```python
from build123d import *

# Parameters (mm, degrees)
SKETCH1_R               = 2
BOSS_EXTRUDE1_DEPTH     = 20
CUT_EXTRUDE1_DEPTH      = 37.932370625
CUT_EXTRUDE1_DEPTH_BACK = 37.932370625
SKETCH2_W               = 20
SKETCH2_H               = 16.5
FILLET1_R               = 4
CHAMFER1_SIZE           = 4
CHAMFER1_SIZE_2         = 11.616843511
SKETCH4_R               = 2.5
CUT_EXTRUDE2_DEPTH      = 40.446165847
CUT_EXTRUDE3_START      = -3
CUT_EXTRUDE3_DEPTH      = 37.446165847


with BuildPart() as part:
    # Sketch1 → Boss-Extrude1 (new, symmetric)
    with BuildSketch(Plane.XY):
        with BuildLine():
            Line((-2.75862069, 2.896551724), (6.8, 12))
            Line((6.8, 12), (30, 12))
            Line((30, 12), (30, 4))
            Line((30, 4), (10, 4))
            Line((10, 4), (2.75862069, -2.896551724))
            ThreePointArc((2.75862069, -2.896551724), (-2.896551724, -2.75862069), (-2.75862069, 2.896551724))
        make_face()
        Circle(SKETCH1_R, mode=Mode.SUBTRACT)
    extrude(amount=BOSS_EXTRUDE1_DEPTH, both=True)

    # Sketch2 → Cut-Extrude1 (cut, two sides: drawn at the far end of the back side and taken through both)
    with BuildSketch(Plane.XZ.offset(-4).offset(-CUT_EXTRUDE1_DEPTH_BACK)):
        with Locations((-2, 16.75)):
            Rectangle(SKETCH2_W, SKETCH2_H)
        with Locations((-2, -16.75)):
            Rectangle(SKETCH2_W, SKETCH2_H)
    extrude(amount=CUT_EXTRUDE1_DEPTH + CUT_EXTRUDE1_DEPTH_BACK, mode=Mode.SUBTRACT)

    # Fillet1
    # the kernel refuses this fillet: 4 mm, written as the material it takes off along each edge
    with BuildSketch(Plane(origin=(8, 2.095238095, -33.4221588), x_dir=(0.7241379310344825, 0.6896551724137934, 0), z_dir=(0, 0, 1))) as fillet1_piece_1:
        with BuildLine():
            CenterArc((6.599216221, 1.129177032), FILLET1_R, 136.397181027, 60)
            Line((3.702664496, 3.887797721), (3.644733462, 3.942970135))
            Line((3.644733462, 3.942970135), (-0.057931034, 0.055172414))
            Line((-0.057931034, 0.055172414), (0, -0.08))
            ThreePointArc((0, -0.08), (1.380952381, -0.08), (2.685158533, -0.022583541))
            Line((2.685158533, -0.022583541), (2.761904762, 0))
        make_face()
    extrude(amount=24.9221588, mode=Mode.SUBTRACT)
    with BuildSketch(Plane(origin=(8, 12, -8.5), x_dir=(0, -1, 0), z_dir=(0, 0, -1))) as fillet1_piece_2:
        with BuildLine():
            CenterArc((FILLET1_R, -FILLET1_R), FILLET1_R, 90, 90)
            Line((0, -FILLET1_R), (-FILLET1_R * 0.02, -FILLET1_R))
            Line((-FILLET1_R * 0.02, -FILLET1_R), (-FILLET1_R * 0.02, FILLET1_R * 0.02))
            Line((-FILLET1_R * 0.02, FILLET1_R * 0.02), (FILLET1_R, FILLET1_R * 0.02))
            Line((FILLET1_R, FILLET1_R * 0.02), (FILLET1_R, 0))
        make_face()
    extrude(amount=21.5, mode=Mode.SUBTRACT)
    with BuildSketch(Plane(origin=(8, 12, 8.5), x_dir=(0, -1, 0), z_dir=(0, 0, 1))) as fillet1_piece_3:
        with BuildLine():
            CenterArc((FILLET1_R, FILLET1_R), FILLET1_R, 180, 90)
            Line((0, FILLET1_R), (-FILLET1_R * 0.02, FILLET1_R))
            Line((-FILLET1_R * 0.02, FILLET1_R), (-FILLET1_R * 0.02, -FILLET1_R * 0.02))
            Line((-FILLET1_R * 0.02, -FILLET1_R * 0.02), (FILLET1_R, -FILLET1_R * 0.02))
            Line((FILLET1_R, -FILLET1_R * 0.02), (FILLET1_R, 0))
        make_face()
    extrude(amount=21.5, mode=Mode.SUBTRACT)
    with BuildSketch(Plane(origin=(8, 2.095238095, 33.4221588), x_dir=(0.7241379310344824, 0.6896551724137936, 0), z_dir=(0, 0, -1))) as fillet1_piece_4:
        with BuildLine():
            CenterArc((6.599216221, -1.129177032), FILLET1_R, 163.602818973, 60)
            Line((3.702664496, -3.887797721), (3.644733462, -3.942970135))
            Line((3.644733462, -3.942970135), (-0.057931034, -0.055172414))
            Line((-0.057931034, -0.055172414), (0, 0.08))
            ThreePointArc((0, 0.08), (1.380952381, 0.08), (2.685158533, 0.022583541))
            Line((2.685158533, 0.022583541), (2.761904762, 0))
        make_face()
    extrude(amount=24.9221588, mode=Mode.SUBTRACT)

    # Chamfer1
    # the kernel refuses this chamfer: 11.616843511, 4 mm, written as the material it adds along each edge
    with BuildSketch(Plane(origin=(12, 8, -8.5), x_dir=(-1, 0, 0), z_dir=(0, -1, 0))) as chamfer1_piece_1_section:
        Polygon((4 + CHAMFER1_SIZE, 0), (4, CHAMFER1_SIZE_2), (4, 0), align=None)
    chamfer1_piece_1 = revolve(axis=Axis((12, 8, -8.5), (0, 0, -1)), revolution_arc=359.64, mode=Mode.PRIVATE)
    chamfer1_piece_1 = split(chamfer1_piece_1, bisect_by=Plane(origin=(6.815559228, 9.673675178, -20), z_dir=(0, 0, 1)), keep=Keep.TOP, mode=Mode.PRIVATE)
    chamfer1_piece_1 = split(chamfer1_piece_1, bisect_by=Plane(origin=(6.815559228, 12, -12.048091189), z_dir=(0, -1, 0)), keep=Keep.TOP, mode=Mode.PRIVATE)
    chamfer1_piece_1 = split(chamfer1_piece_1, bisect_by=Plane(origin=(5.646379541, 10.901313849, -12.048091189), z_dir=(0.6896551724137935, -0.7241379310344824, 0)), keep=Keep.TOP, mode=Mode.PRIVATE)
    chamfer1_piece_1 = split(chamfer1_piece_1, bisect_by=Plane(origin=(11.163620921, 5.1082104, -12.048091189), z_dir=(-0.6896551724137935, 0.7241379310344825, 0)), keep=Keep.TOP, mode=Mode.PRIVATE)
    add(chamfer1_piece_1)
    with BuildSketch(Plane(origin=(8, 7.464101615, -8.5), x_dir=(-0.9944459243087849, 0, 0.10524877018591122), z_dir=(0, 1, 0))) as chamfer1_piece_2_section:
        Polygon((CHAMFER1_SIZE * 0.994445924309, -CHAMFER1_SIZE * 0.105248770186), (-CHAMFER1_SIZE_2 * 0.105248770183, -CHAMFER1_SIZE_2 * 0.994445924283), (0, 0), align=None)
    chamfer1_piece_2 = extrude(amount=0.535898385, mode=Mode.PRIVATE)
    chamfer1_piece_2 = split(chamfer1_piece_2, bisect_by=Plane(origin=(6.666533122, 7.732050808, -20), z_dir=(0, 0, 1)), keep=Keep.TOP, mode=Mode.PRIVATE)
    add(chamfer1_piece_2)
    with BuildSketch(Plane(origin=(12, 7.464101615, -8.5), x_dir=(-1, 0, 0), z_dir=(0, 1, 0))) as chamfer1_piece_3_section:
        Polygon((4 + CHAMFER1_SIZE, 0), (4, -CHAMFER1_SIZE_2), (4, 0), align=None)
    chamfer1_piece_3 = revolve(axis=Axis((12, 7.464101615, -8.5), (0, 0, 1)), revolution_arc=359.64, mode=Mode.PRIVATE)
    chamfer1_piece_3 = split(chamfer1_piece_3, bisect_by=Plane(origin=(6.73533338, 5.888138527, -20), z_dir=(0, 0, 1)), keep=Keep.TOP, mode=Mode.PRIVATE)
    chamfer1_piece_3 = split(chamfer1_piece_3, bisect_by=Plane(origin=(6.73533338, 12, -12.010330429), z_dir=(0, -1, 0)), keep=Keep.TOP, mode=Mode.PRIVATE)
    chamfer1_piece_3 = split(chamfer1_piece_3, bisect_by=Plane(origin=(3.713793343, 9.060755565, -12.010330429), z_dir=(0.6896551724137935, -0.7241379310344824, 0)), keep=Keep.TOP, mode=Mode.PRIVATE)
    chamfer1_piece_3 = split(chamfer1_piece_3, bisect_by=Plane(origin=(9.231034723, 3.267652117, -12.010330429), z_dir=(-0.6896551724137935, 0.7241379310344825, 0)), keep=Keep.TOP, mode=Mode.PRIVATE)
    add(chamfer1_piece_3)
    with BuildSketch(Plane(origin=(12, 8, 8.5), x_dir=(-0.9999802608561372, -0.006283143965558626, 0), z_dir=(-0.006283143965558626, 0.9999802608561372, 0))) as chamfer1_piece_4_section:
        Polygon((-4, CHAMFER1_SIZE_2), (-4 - CHAMFER1_SIZE, 0), (-4, 0), align=None)
    chamfer1_piece_4 = revolve(axis=Axis((12, 8, 8.5), (0, 0, 1)), revolution_arc=359.64, mode=Mode.PRIVATE)
    chamfer1_piece_4 = split(chamfer1_piece_4, bisect_by=Plane(origin=(8.929227056, 11.070772944, 20), z_dir=(0, 0, -1)), keep=Keep.TOP, mode=Mode.PRIVATE)
    chamfer1_piece_4 = split(chamfer1_piece_4, bisect_by=Plane(origin=(8.929227056, 12, 13.636607489), z_dir=(0, -1, 0)), keep=Keep.TOP, mode=Mode.PRIVATE)
    chamfer1_piece_4 = split(chamfer1_piece_4, bisect_by=Plane(origin=(7.452453946, 12.62138471, 13.636607489), z_dir=(0.6896551724137935, -0.7241379310344824, 0)), keep=Keep.TOP, mode=Mode.PRIVATE)
    chamfer1_piece_4 = split(chamfer1_piece_4, bisect_by=Plane(origin=(12.969695325, 6.828281262, 13.636607489), z_dir=(-0.6896551724137935, 0.7241379310344825, 0)), keep=Keep.TOP, mode=Mode.PRIVATE)
    add(chamfer1_piece_4)
    with BuildSketch(Plane(origin=(8, 8, 8.5), x_dir=(0.012547158200392034, 0, 0.9999212813122313), z_dir=(0, -1, 0))) as chamfer1_piece_5_section:
        Polygon((CHAMFER1_SIZE_2 * 0.999921281287, CHAMFER1_SIZE_2 * 0.0125471582001), (-CHAMFER1_SIZE * 0.0125471582004, CHAMFER1_SIZE * 0.999921281312), (0, 0), align=None)
    chamfer1_piece_5 = extrude(amount=0.535898385, mode=Mode.PRIVATE)
    chamfer1_piece_5 = split(chamfer1_piece_5, bisect_by=Plane(origin=(6.666533122, 7.732050808, 20), z_dir=(0, 0, -1)), keep=Keep.TOP, mode=Mode.PRIVATE)
    add(chamfer1_piece_5)
    with BuildSketch(Plane(origin=(12, 7.464101615, 8.5), x_dir=(-0.9999802608561402, 0.006283143965082117, 0), z_dir=(-0.006283143965082117, -0.9999802608561402, 0))) as chamfer1_piece_6_section:
        Polygon((-4, -CHAMFER1_SIZE_2), (-4 - CHAMFER1_SIZE, 0), (-4, 0), align=None)
    chamfer1_piece_6 = revolve(axis=Axis((12, 7.464101615, 8.5), (0, 0, -1)), revolution_arc=359.64, mode=Mode.PRIVATE)
    chamfer1_piece_6 = split(chamfer1_piece_6, bisect_by=Plane(origin=(8.748719475, 3.446621368, 20), z_dir=(0, 0, -1)), keep=Keep.TOP, mode=Mode.PRIVATE)
    chamfer1_piece_6 = split(chamfer1_piece_6, bisect_by=Plane(origin=(8.748719475, 12, 12.595227268), z_dir=(0, -1, 0)), keep=Keep.TOP, mode=Mode.PRIVATE)
    chamfer1_piece_6 = split(chamfer1_piece_6, bisect_by=Plane(origin=(3.55025715, 8.905006809, 12.595227268), z_dir=(0.6896551724137935, -0.7241379310344824, 0)), keep=Keep.TOP, mode=Mode.PRIVATE)
    chamfer1_piece_6 = split(chamfer1_piece_6, bisect_by=Plane(origin=(9.067498529, 3.111903361, 12.595227268), z_dir=(-0.6896551724137935, 0.7241379310344825, 0)), keep=Keep.TOP, mode=Mode.PRIVATE)
    add(chamfer1_piece_6)

    # Sketch4 → Cut-Extrude2 (cut, through all)
    with BuildSketch(Plane(origin=(0, 12, 0), x_dir=(1, 0, 0), z_dir=(0, 1, 0))):
        with Locations(Location((20.715624268, -10, 0), (0, 0, 180))):
            Circle(SKETCH4_R)
    cut_extrude2 = extrude(amount=-CUT_EXTRUDE2_DEPTH, mode=Mode.SUBTRACT)

    # Sketch5 → Cut-Extrude3 (cut, through all)
    with BuildSketch(Plane(origin=(0, 12, 0), x_dir=(1, 0, 0), z_dir=(0, 1, 0)).offset(CUT_EXTRUDE3_START)):
        Polygon((20.715624268, -14.330127019), (24.465624268, -12.165063509), (24.465624268, -7.834936491), (20.715624268, -5.669872981), (16.965624268, -7.834936491), (16.965624268, -12.165063509), align=None)
    cut_extrude3 = extrude(amount=-CUT_EXTRUDE3_DEPTH, mode=Mode.SUBTRACT)

    # Mirror1: Cut-Extrude2, Cut-Extrude3 across plane
    add(cut_extrude2.mirror(Plane.XY), mode=Mode.SUBTRACT)
    add(cut_extrude3.mirror(Plane.XY), mode=Mode.SUBTRACT)


solid = part.part
```
Input: part model. Units: mm. Frame: model coordinates. A direction names the side the tool comes from. Give positions to 0.01 mm unless a question says otherwise; leave off trailing zeros. Order: outer loops, then holes, each group sorted by start corner. A loop starts at its lowest first (then second) coordinate and runs counter-clockwise, first axis right, second up.
1. Pin query (flat end, axial travel): pin 1 (8 mm diameter, centred on x = 2, y = -1, fed in from +Z); pin 2 (6 mm diameter, centred on x = 19.5, z = 8.5, fed in from -Y); pin 3 (6 mm diameter, centred on x = 5, z = 8, fed in from -Y). Return the tip coordinate at first contact, or that it passes through.
Derived:
pin 1: stops at z = 8.5
pin 2: stops at y = 4
pin 3: stops at y = -3.46
2. Section D-D on x = 0. Return the cut outline in (y, z), and give its area (3 significant figures).
Derived:
outline: (-4, -8.5) - (-2, -8.5) - (-2, 8.5) - (-4, 8.5) - close; (2, -8.5) - (5.52, -8.5) - (5.52, 8.5) - (2, 8.5) - close
area: 93.9 mm2
3. Section A-A on y = -1.5. Return the cut outline in (x, z) (3 decimals), and give its area (3 significant figures).
Derived:
outline: (-3.708, -8.5) - (-1.323, -8.5) - (-1.323, 8.5) - (-3.708, 8.5) - close; (1.323, -8.5) - (4.225, -8.5) - (4.225, 8.5) - (1.323, 8.5) - close
area: 89.9 mm2
4. Mould query, pull axis Z, two halves, no side actions, for faces 1 (the flat face through (5.952, 7.728, -14.17)), 2 (the flat face through (18.81, 6.54, -13.23)), 3 (the cylindrical face through (-2.835, -2.822, 0.119)). Classes: released by +Z, released by -Z, zero draft, split by the parting line, or undercut.
Derived:
face 1: released by -Z
face 2: undercut
face 3: zero draft
5. Reachability of faces 4 (the flat face through (30, 8, 0)), 5 (the flat face through (22.564, 6.535, 13.263)) from +Z, -Z, +X, -X, +Y, -Y: full face, straight path, thin tool, end or side. Return the list, or none.
Derived:
face 4: +Z, -Z, +X, +Y, -Y
face 5: -Y
6. Material intervals for L1, parallel to Z at x = 20.5, y = 6; L2, parallel to Z at x = 19.5, y = 11; L3, parallel to Z at x = 1, y = 4.5, sorted ascending.
Derived:
L1: z = -20 to -14.21, -5.79 to 5.79, 14.21 to 20
L2: z = -20 to -12.18, -7.82 to 7.82, 12.18 to 20
L3: z = -8.5 to 8.5
7. Section B-B on x = 22.5. Return the cut outline in (y, z), and give its area (3 significant figures).
Derived:
outline: (4, -20) - (12, -20) - (12, -11.75) - (9, -11.75) - (9, -13.3) - (4, -13.3) - close; (4, -6.7) - (9, -6.7) - (9, -8.25) - (12, -8.25) - (12, 8.25) - (9, 8.25) - (9, 6.7) - (4, 6.7) - close; (4, 13.3) - (9, 13.3) - (9, 11.75) - (12, 11.75) - (12, 20) - (4, 20) - close
area: 233 mm2
8. Section C-C on z = 10. Return the cut outline in (x, y), and give its area (3 significant figures).
Derived:
outline: (4.52, 7.46) arc R7.48 ccw to (7.42, 1.54) - (10, 4) - (16.97, 4) - (16.97, 9) - (18.22, 9) - (18.22, 12) - (6.8, 12) - (4.82, 10.12) arc R7.48 ccw to (4.52, 8) - close; (23.22, 9) - (24.47, 9) - (24.47, 4) - (30, 4) - (30, 12) - (23.22, 12) - close
area: 154 mm2
